from build123d import *

# Parameters (mm, degrees)
F1_DEPTH = 30
F3_D     = 6.7
F3_DEPTH = 20
F3_TIP   = 2.0128830737
F5_D     = 14
F7_D     = 8.5


with BuildPart() as f1:
    # F0 (on Front) → F1 (new body)
    with BuildSketch(Plane.XZ):
        Polygon((-14, 20), (14, 20), (14, -20), (44, -20), (44, 50), (-44, 50), (-44, -20), (-14, -20), align=None)
    extrude(amount=F1_DEPTH)

    # F3
    with Locations(Plane(origin=(-44, 0, 0), x_dir=(0, -1, 0), z_dir=(-1, 0, 0))):
        with Locations((15, 40), (15, 25)):
            Hole(F3_D / 2, depth=F3_DEPTH)
            with Locations((0, 0, -(F3_DEPTH + F3_TIP / 2))):  # 118° drill point
                Cone(0, F3_D / 2, F3_TIP, mode=Mode.SUBTRACT)

    # F5 (through all)
    with Locations(Plane.XY.offset(50)):
        with Locations((0, -15)):
            Hole(F5_D / 2)

    # F7 (through all)
    with Locations(Plane(origin=(-44, 0, 0), x_dir=(0, -1, 0), z_dir=(-1, 0, 0))):
        with Locations((15, 0)):
            Hole(F7_D / 2)


solid = f1.part
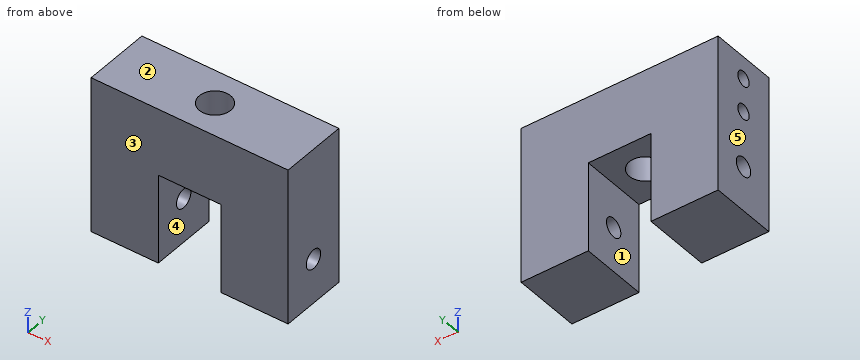
For this review, take the finished solid that the model builds, in its own axes (mm). Face numbers are marked on the shaded views. A direction names the side the tool comes from. Round coordinates to 2 decimals unless told otherwise and drop trailing zeros. Write each loop counter-clockwise with the first axis right and the second up, starting at its lowest first coordinate (ties: lowest second). Pieces come first, ordered by that corner, then holes. Notation, with made-up numbers: (73, -13) -> (112, -13) arc R23 ccw to (112, 9) -> close; hole circle Ø1 at (57.5, -9.5). An arc over 180 degrees is marked (long way). Put each result on its own line as item: value.
Q1. Consider section A-A on z = 12.5. State the section outline as (x, y) points.
Determined:
outline: (-44, -30) -> (-14, -30) -> (-14, 0) -> (-44, 0) -> close; (14, -30) -> (44, -30) -> (44, 0) -> (14, 0) -> close
Q2. Consider section D-D on x = -16. State the section outline as (y, z) points.
Determined:
outline: (-30, -20) -> (0, -20) -> (0, 50) -> (-30, 50) -> close; hole circle Ø8.5 at (-15, 0)
Q3. The part is to be moulded in two halves that separate along X. For the marked faces 3, 4 and 5, say which applies: released by +X, released by -X, zero draft, split by the parting line, or undercut.
Determined:
face 3: zero draft
face 4: undercut
face 5: released by -X
Q4. To check wall thickness, follow L1, parallel to Z at x = -33, y = -15; L2, parallel to X at y = -8.25, z = -5; L3, parallel to Y at x = 0, z = 20.5. State the ranges of each line that lie inside material, in increasing order. Write a range as [from, to].
Determined:
L1: z = [-20, -4.25], [4.25, 21.65], [28.35, 36.65], [43.35, 50]
L2: x = [-44, -14], [14, 44]
L3: y = [-30, -22], [-8, 0]
Q5. Clearance check with flat-ended pins moving along their axes: pin 1 Ø13.5 at (y, z) = (-15, 0) entering from -X; pin 2 Ø11 at (x, y) = (0, -15) entering from +Z; pin 3 Ø8.5 at (x, y) = (-4.5, -11) entering from -Z. State where each tip first meets the part, or that it passes through.
Determined:
pin 1: stops at x = -44
pin 2: passes through
pin 3: stops at z = 20
Q6. Machinability: for the marked faces 1 and 2, which of the approach directions +Z, -Z, +X, -X, +Y, -Y give a long, thin tool a straight path to every point of the face, cutting with its end or side? Answer none if there is none.
Determined:
face 1: -Z, +Y, -Y
face 2: +Z, +X, -X, +Y, -Y
Q7. Consider section B-B on x = -1. State the section outline as (y, z) points, and give its area (3 significant figures).
Determined:
outline: (-30, 20) -> (-21.93, 20) -> (-21.93, 50) -> (-30, 50) -> close; (-8.07, 20) -> (0, 20) -> (0, 50) -> (-8.07, 50) -> close
area: 484 mm^2
Q8. Consider section C-C on z = 0. State the section outline as (x, y) points.
Determined:
outline: (-44, -30) -> (-14, -30) -> (-14, -19.25) -> (-44, -19.25) -> close; (-44, -10.75) -> (-14, -10.75) -> (-14, 0) -> (-44, 0) -> close; (14, -30) -> (44, -30) -> (44, -19.25) -> (14, -19.25) -> close; (14, -10.75) -> (44, -10.75) -> (44, 0) -> (14, 0) -> close
